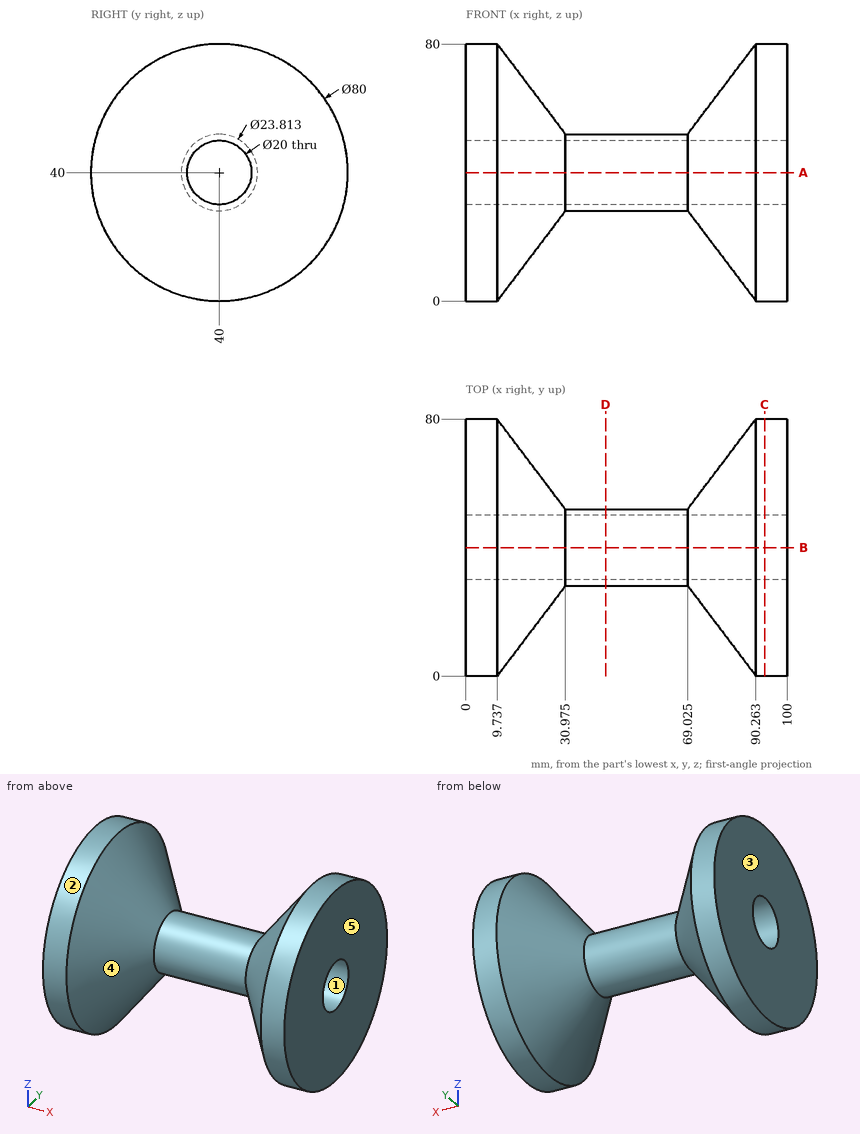
Answer from the drawing. Dimensions are ordinates in mm from the lowest x, y and z of the part. A direction names the side the tool comes from. Coordinates: 2 decimals unless noted, no trailing zeros. Loops run counter-clockwise (first coordinate to the right, second up) from the corner with the lowest first, then second, coordinate; pieces in that order, holes last. Notation, with made-up numbers: (-32.5, 79.5) -> (24.5, 79.5) arc R23 cw to (24.5, 87.5) -> close; hole circle Ø2 at (2.25, 79.25). An arc over 180 degrees is marked (long way). Answer in a Markdown table with one row per item.
Item 1: A cutting plane is placed at C-C on x = 93. Determine the outline of the cut face in (y, z), plus the area to 3 significant figures.
Returned:
| item | result |
|---|---|
| outline | circle Ø80 at (40, 40); hole circle Ø20 at (40, 40) |
| area | 4,710 mm^2 |
Item 2: Straight lines are drawn through the part: line 1 along Y through (x, z) = (39, 40); line 2 along Y through (x, z) = (83, 48); line 3 along X through (y, z) = (72, 17.5). For each, find the intervals that lie inside material, in ascending order. Write a range as [from, to].
Returned:
| item | result |
|---|---|
| line 1 | y = [28.09, 30], [50, 51.91] |
| line 2 | y = [10.68, 34], [46, 69.32] |
| line 3 | x = [0, 10.4], [89.6, 100] |
Item 3: A cutting plane is placed at D-D on x = 43.5. Determine the outline of the cut face in (y, z), plus the area to 3 significant figures.
Returned:
| item | result |
|---|---|
| outline | circle Ø23.81 at (40, 40); hole circle Ø20 at (40, 40) |
| area | 131 mm^2 |
Item 4: Each of these flat-tipped pins is pushed along its axis until it touches: P1, Ø1, axis at x = 82, y = 28, coming from the +Z side (1 decimal); P2, Ø5, axis at x = 13.5, y = 17.5, coming from the -Z side; P3, Ø2, axis at x = 35.5, z = 32, coming from the +Y side. Where does it stop, or does it pass through?
Returned:
| item | result |
|---|---|
| P1 | stops at z = 67.2 |
| P2 | stops at z = 8.6 |
| P3 | stops at y = 49.63 |
Item 5: For a pull along Y with two mould halves and no side action, classify the marked faces 1, 2 and 3 as released by +Y, released by -Y, zero draft, split by the parting line, or undercut.
Returned:
| item | result |
|---|---|
| face 1 | undercut |
| face 2 | split by the parting line |
| face 3 | zero draft |
Item 6: A cutting plane is placed at A-A on z = 40. Determine the outline of the cut face in (x, y) (1 decimal).
Returned:
| item | result |
|---|---|
| outline | (0, 0) -> (9.7, 0) -> (31, 28.1) -> (69, 28.1) -> (90.3, 0) -> (100, 0) -> (100, 30) -> (0, 30) -> close; (0, 50) -> (100, 50) -> (100, 80) -> (90.3, 80) -> (69, 51.9) -> (31, 51.9) -> (9.7, 80) -> (0, 80) -> close |
Item 7: For the marked faces 4 and 5, determine the directions among +Z, -Z, +X, -X, +Y, -Y from which every point of the face is accessible in a straight line to the end or side of a thin tool.
Returned:
| item | result |
|---|---|
| face 4 | none |
| face 5 | +Z, -Z, +X, +Y, -Y |
